Can you work these out from the model? Positions are in its coordinate system, mm. A direction names the side the tool comes from. Coordinates: 2 decimals unless noted, no trailing zeros. Loops run counter-clockwise (first coordinate to the right, second up) from the corner with the lowest first, then second, coordinate; pieces in that order, holes last. Notation, with made-up numbers: (72.5, 5.25) -> (104.5, 5.25) arc R19 cw to (104.5, 29.25) -> close; hole circle Ø3 at (49, 65.5). An arc over 180 degrees is marked (long way). Use one line per item in the form item = value. Start each with the question number.
(1) I need wall thicknesses on line 1 (Z direction, x = -50.5, y = -19.5); line 2 (Z direction, x = -14, y = -12); line 3 (X direction, y = -1.5, z = 27.5). Which ranges of each line are inside material? Lowest first, please. Write a range as [from, to].
(2) I'm going to push flat-ended pins straight in: pin 1 (1 mm diameter, centred on y = -19.5, z = 30.5, fed in from -X); pin 2 (3.5 mm diameter, centred on x = -49, z = 28.5, fed in from -Y); pin 3 (6 mm diameter, centred on x = -48, z = 11, fed in from -Y). Where does each tip first touch, or does it pass through?
(3) Imagine slicing it at B-B (z = 27). List the corners of the cut face in (x, y) for me, plus the area to 4 significant figures.
(4) Imagine slicing it at D-D (x = -9). List the corners of the cut face in (y, z) for me.
(5) On a 3-axis mill with a long thin cutter (end or side, diameter ignored), from which of +Z, -Z, +X, -X, +Y, -Y can I reach the whole of each face in a straight line? I mean faces 1 (the flat face through (-39, -20, 13)), 2 (the cylindrical face through (-59.493, -10.657, 10.357)), 3 (the flat face through (-60, -11, 8)). Say none if no direction works.
(6) Thinking about a two-plate mould opening in Z: for faces 4 (the flat face through (-15, -27, 27)), 5 (the flat face through (-48, -10, 41.1)), 6 (the cylindrical face through (-4.03, -23.96, 30.45)), 7 (the flat face through (-49, -20, 34.383)), which applies, released by +Z, released by -Z, zero draft, split by the parting line, or undercut?
(7) Imagine slicing it at A-A (x = -15). List the corners of the cut face in (y, z) for me, plus the area to 3 significant figures.
(8) Imagine slicing it at C-C (y = -25). List the corners of the cut face in (x, z) for me, plus the area to 3 significant figures.
```python
from build123d import *

# Parameters (mm, degrees)
F0_W      = 59
F0_H      = 41
F1_DEPTH  = 21
F2_R      = 11.5
F3_DEPTH  = 6
F2_W      = 11
F2_H      = 15
F4_DEPTH  = 2
F2_R_2    = 5.5
F5_DEPTH  = 2
F2_R_3    = 2.5
F7_DEPTH  = 1
F8_R      = 2.913941294
F9_DEPTH  = 1
F10_R     = 7.1742199979
F11_DEPTH = 0.1


# Not quite as in the source:
# - a fillet or chamfer that OpenCascade refuses, or shapes differently, is made with other operations: its cross-section is extruded or revolved along the edge and cut away or added
# - a feature of the source that left no trace in its solid (it failed there, or was rolled back) is left out


with BuildPart() as f1:
    # F0 (on Front) → F1 (new body)
    with BuildSketch(Plane.XZ):
        with Locations((-29.5, 20.5)):
            Rectangle(F0_W, F0_H)
    extrude(amount=F1_DEPTH)

    # F2 (on face) → F3 (join)
    with BuildSketch(Plane.XZ.offset(21)):
        with Locations((-15, 27)):
            Circle(F2_R)
    extrude(amount=F3_DEPTH)

    # F2 (on face) → F4 (cut)
    with BuildSketch(Plane.XZ.offset(21)):
        with Locations((-49.2600723803, 26.8833857775)):
            Rectangle(F2_W, F2_H)
    extrude(amount=-F4_DEPTH, mode=Mode.SUBTRACT)

    # F2 (on face) → F5 (join)
    with BuildSketch(Plane.XZ.offset(21)):
        with Locations((-49.2600723803, 9.5262574032)):
            Circle(F2_R_2)
    extrude(amount=F5_DEPTH)

    # F6: fillet of radius 3 on 1 edges, made by hand

    # F6_s1 → F6_t2 (revolve, cut)
    with BuildSketch(Plane.XY.offset(9.5262574032)):
        with BuildLine():
            ThreePointArc((-43.7600723803, -21), (-44.8564486975, -22.4494897428), (-46.5884995051, -23))
            Line((-46.5884995051, -23), (-43.7600723803, -23))
            Line((-43.7600723803, -23), (-43.7600723803, -21))
        make_face()
    revolve(axis=Axis((-49.2600723803, -23, 9.5262574032), (0, -1, 0)), mode=Mode.SUBTRACT)

    # F2 (on face) → F7 (cut)
    with BuildSketch(Plane.XZ.offset(21)):
        with Locations((-39.2693579197, 13.1571451202)):
            Circle(F2_R_3)
        with Locations((-39.2693579197, 6.7239077762)):
            Circle(F2_R_3)
    extrude(amount=-F7_DEPTH, mode=Mode.SUBTRACT)

    # F8 (on face) → F9 (join)
    with BuildSketch(Plane(origin=(-59, 0, 0), x_dir=(0, -1, 0), z_dir=(-1, 0, 0))):
        with Locations((11.0362954438, 7.4682990089)):
            Circle(F8_R)
    extrude(amount=F9_DEPTH)

    # F10 (on face) → F11 (join)
    with BuildSketch(Plane.XY.offset(41)):
        with Locations((-47.7264709771, -10.5)):
            Circle(F10_R)
    extrude(amount=F11_DEPTH)


solid = f1.part
```
Worked out:
q1.line_1 = [0, 19.38], [34.38, 41]
q1.line_2 = [0, 41]
q1.line_3 = [-59, 0]
q2.pin_1 = -59
q2.pin_2 = -19
q2.pin_3 = -23
q3.outline = (-59, -21) -> (-54.76, -21) -> (-54.76, -19) -> (-43.76, -19) -> (-43.76, -21) -> (-26.5, -21) -> (-26.5, -27) -> (-3.5, -27) -> (-3.5, -21) -> (0, -21) -> (0, 0) -> (-59, 0) -> close
q3.area = 1,355 mm2
q4.outline = (-27, 17.19) -> (-21, 17.19) -> (-21, 0) -> (0, 0) -> (0, 41) -> (-21, 41) -> (-21, 36.81) -> (-27, 36.81) -> close
q5.face_1 = -Y
q5.face_2 = -X
q5.face_3 = +Z, -Z, -X, +Y, -Y
q6.face_4 = zero draft
q6.face_5 = released by +Z
q6.face_6 = split by the parting line
q6.face_7 = undercut
q7.outline = (-27, 15.5) -> (-21, 15.5) -> (-21, 0) -> (0, 0) -> (0, 41) -> (-21, 41) -> (-21, 38.5) -> (-27, 38.5) -> close
q7.area = 999 mm2
q8.outline = circle Ø23 at (-15, 27)
q8.area = 415 mm2
